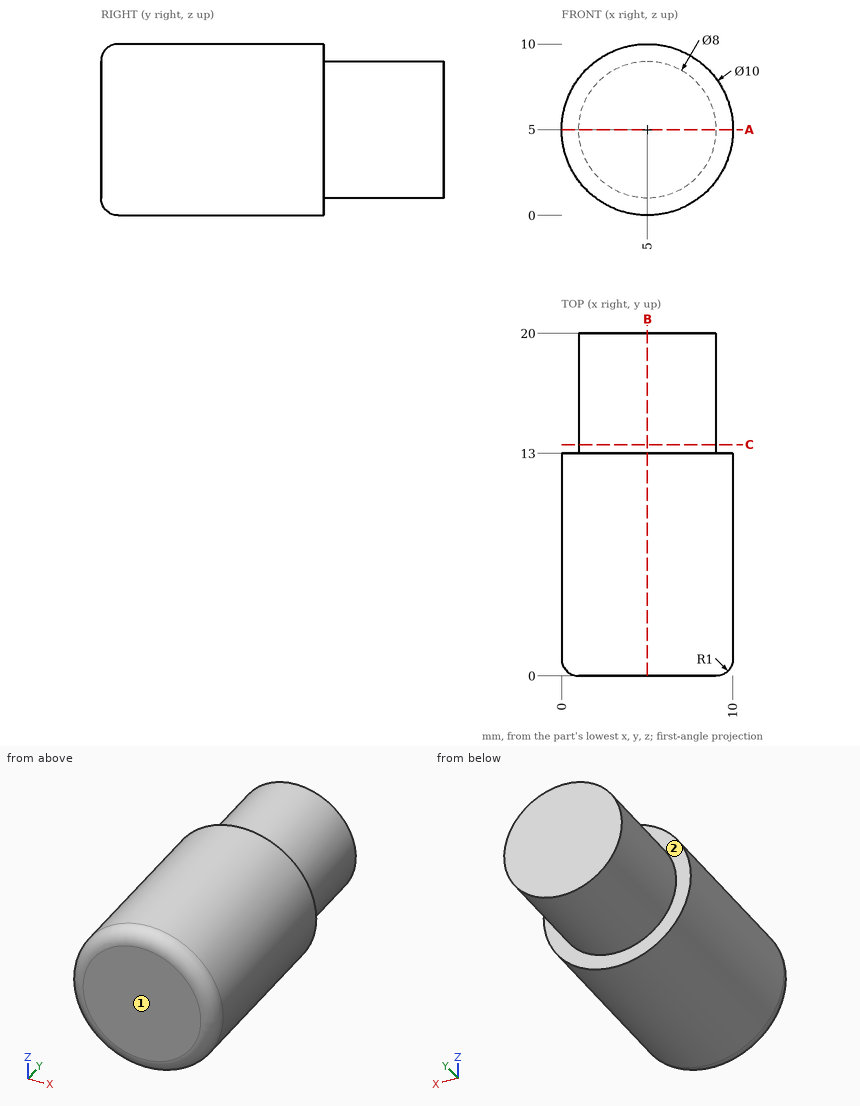
Input: dimensioned drawing with shaded views. Units: mm. Origin: part minimum x, y, z. A direction names the side the tool comes from. Coordinates: 2 decimals unless noted, no trailing zeros. Loops run counter-clockwise (first coordinate to the right, second up) from the corner with the lowest first, then second, coordinate; pieces in that order, holes last. Notation, with made-up numbers: M 84.5,-25 L 110.5,-25 A10 ccw 110.5,-16 Z; hole C 18.5,76 d2. An arc over 180 degrees is marked long. Use a Markdown table: item, result. Add a question column.
1) Set-up query: the marked faces 1 and 2. Return all of +Z, -Z, +X, -X, +Y, -Y with unobstructed straight access to the full face (end or side cutting, diameter ignored); none if empty.
2) Section C-C, the plane y = 13.5. Return the cut outline in (x, z), plus the area to 3 significant figures.
3) Pin query (flat end, axial travel): P1, Ø1.5, axis at x = 7, y = 17, coming from the +Z side; P2, Ø3, axis at y = 16.5, z = 6.5, coming from the -X side; P3, Ø4, axis at x = 7.5, y = 12, coming from the +Z side. Return the tip coordinate at first contact, or that it passes through.
4) Section A-A, the plane z = 5. Return the cut outline in (x, y).
5) Line query: L1, parallel to X at y = 15.75, z = 5; L2, parallel to Z at x = 2.5, y = 1.5; L3, parallel to Y at x = 1.5, z = 1.5. Output: solid intervals per line, ascending. Write a range as from..to.
6) Section B-B, the plane x = 5. Return the cut outline in (y, z).
Answer below:
| question | item | result |
|---|---|---|
| 1 | face 1 | +Z, -Z, +X, -X, -Y |
| 1 | face 2 | +Y |
| 2 | outline | C 5,5 d8 |
| 2 | area | 50.3 mm2 |
| 3 | P1 | z = 8.8 |
| 3 | P2 | x = 1 |
| 3 | P3 | z = 9.97 |
| 4 | outline | M 0,1 A1 ccw 1,0 L 9,0 A1 ccw 10,1 L 10,13 L 9,13 L 9,20 L 1,20 L 1,13 L 0,13 Z |
| 5 | L1 | 1..9 |
| 5 | L2 | 0.67..9.33 |
| 5 | L3 | 0.69..13 |
| 6 | outline | M 0,1 A1 ccw 1,0 L 13,0 L 13,1 L 20,1 L 20,9 L 13,9 L 13,10 L 1,10 A1 ccw 0,9 Z |
